```python
from build123d import *

# Parameters (mm, degrees)
BOSS_EXTRUDE3_DEPTH                           = 12.7
BOSS_EXTRUDE4_DEPTH                           = 38.1
CBORE_FOR_M3_PAN_HEAD_MACHINE_SCREW1_AT_COUNT = 2
CBORE_FOR_M3_PAN_HEAD_MACHINE_SCREW1_AT_PITCH = 66.51875294
CBORE_FOR_M3_PAN_HEAD_MACHINE_SCREW1_2_COUNT  = 2
CBORE_FOR_M3_PAN_HEAD_MACHINE_SCREW1_2_PITCH  = 66.51875294


with BuildPart() as part:
    # Sketch1 → Boss-Extrude3 (new body)
    with BuildSketch(Plane(origin=(0, 0, 0), x_dir=(0, 0, -1), z_dir=(1, 0, 0))):
        with BuildLine():
            Line((38.1, -76.2), (38.1, 0))
            ThreePointArc((38.1, 0), (0, 38.1), (-38.1, 0))
            Line((-38.1, 0), (-38.1, -76.2))
            Line((-38.1, -76.2), (38.1, -76.2))
        make_face()
    extrude(amount=BOSS_EXTRUDE3_DEPTH)

    # Sketch5 → Boss-Extrude4 (add)
    with BuildSketch(Plane(origin=(12.7, 0, 0), x_dir=(0, 0, -1), z_dir=(1, 0, 0))):
        with BuildLine():
            ThreePointArc((-20.358389677, 0), (0, 20.358389677), (20.358389677, 0))
            Line((20.358389677, 0), (38.1, 0))
            ThreePointArc((38.1, 0), (0, 38.1), (-38.1, 0))
            Line((-38.1, 0), (-20.358389677, 0))
        make_face()
    extrude(amount=BOSS_EXTRUDE4_DEPTH)

    # Sketch8 → CBORE for M3 Pan Head Machine Screw1 (revolve, cut)
    with BuildSketch(Plane(origin=(12.7, 0, 0), x_dir=(0, 0, -1), z_dir=(0, 1, 0))):
        Polygon((0, 0), (0, 12.7), (1.7, 12.7), (1.7, 2.4), (3.5, 2.4), (3.5, 0.025), (3.525, 0), align=None)
    cbore_for_m3_pan_head_machine_screw1 = revolve(axis=Axis((19.05, 0, 0), (-1, 0, 0)), mode=Mode.SUBTRACT)

    # CBORE for M3 Pan Head Machine Screw1 at: CBORE for M3 Pan Head Machine Screw1 ×2
    with Locations(*[Vector(0, -0.924225465, 0.381847207) * (i * CBORE_FOR_M3_PAN_HEAD_MACHINE_SCREW1_AT_PITCH) for i in range(1, CBORE_FOR_M3_PAN_HEAD_MACHINE_SCREW1_AT_COUNT)]):
        add(cbore_for_m3_pan_head_machine_screw1, mode=Mode.SUBTRACT)

    # CBORE for M3 Pan Head Machine Screw1 2: CBORE for M3 Pan Head Machine Screw1 ×2
    with Locations(*[Vector(0, -0.924225465, -0.381847207) * (i * CBORE_FOR_M3_PAN_HEAD_MACHINE_SCREW1_2_PITCH) for i in range(1, CBORE_FOR_M3_PAN_HEAD_MACHINE_SCREW1_2_COUNT)]):
        add(cbore_for_m3_pan_head_machine_screw1, mode=Mode.SUBTRACT)


solid = part.part
```
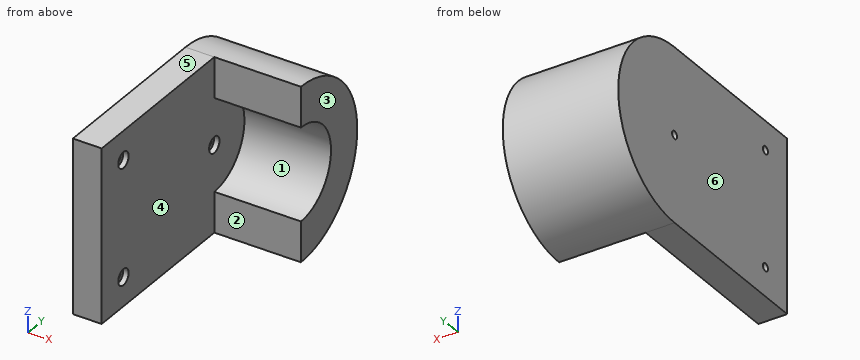
CAD build for the part. Positions are in the model's coordinates, mm. Face numbers are marked on the shaded views. A direction names the side the tool comes from. Coordinates: 2 decimals unless noted, no trailing zeros. Write each loop counter-clockwise with the first axis right and the second up, starting at its lowest first coordinate (ties: lowest second). Pieces come first, ordered by that corner, then holes. Notation, with made-up numbers: (-5.5, 65.5) -> (14.5, 65.5) arc R30 ccw to (14.5, 89.5) -> close; hole circle Ø3 at (3, 72). An arc over 180 degrees is marked (long way). Return JSON: item names as keys, results as strings. Group by question number.
Q1. Which spindle directions (+Z, -Z, +X, -X, +Y, -Y) get a long thin tool onto all of the face, cutting with end or side? Do the marked faces 1, 2 and 3. Say none if no direction does.
Q2. Cut at D-D, the plane z = -25.4. Give the cut face in (x, y) (3 decimals), then the cut area to 3 significant figures.
Q3. Cut at B-B, the plane y = 10.5. Give the cut face in (x, z).
Q4. Cut at C-C, the plane x = 4.5. Give the cut face in (y, z), then the cut area to 3 significant figures.
Q5. Flat gauge pins, fed straight in: pin 1 (4 mm diameter, centred on y = -46.5, z = -18, fed in from +X); pin 2 (3.5 mm diameter, centred on y = -60.5, z = 25.5, fed in from +X); pin 3 (8 mm diameter, centred on y = -61.48, z = -25.4, fed in from -X); pin 4 (14 mm diameter, centred on x = 34, z = -25, fed in from -Y). Where does each tip first touch, or does it go through?
Q6. Drill centre lines: line 1 (Z direction, x = 5, y = 0); line 2 (X direction, y = -41.5, z = -11.5); line 3 (Z direction, x = 10, y = -62.5). Where is each one in solid material? Low to high.
Q7. Pull direction X, two halves, no side cores. Call the marked faces 4, 5 and 6: released by +X, released by -X, zero draft, split by the parting line, or undercut.
Q8. Cut at A-A, the plane z = 0. Give the cut face in (x, y) (3 decimals).
Returned:
{
 "1": {"face 1": "+X, -Y", "face 2": "+Z, -Z, +X, -Y", "face 3": "+Z, -Z, +X, +Y, -Y"},
 "2": {"outline": "(0, -76.2) -> (12.7, -76.2) -> (12.7, -65.003) -> (12.675, -64.978) -> (10.3, -64.978) -> (10.3, -63.178) -> (0, -63.178) -> close; (0, -59.778) -> (10.3, -59.778) -> (10.3, -57.978) -> (12.675, -57.978) -> (12.7, -57.953) -> (12.7, 0) -> (50.8, 0) -> (50.8, 28.398) -> (0, 28.398) -> close", "area": "2,360 mm2"},
 "3": {"outline": "(0, -36.62) -> (50.8, -36.62) -> (50.8, -17.44) -> (12.7, -17.44) -> (12.7, 17.44) -> (50.8, 17.44) -> (50.8, 36.62) -> (0, 36.62) -> close"},
 "4": {"outline": "(-76.2, -38.1) -> (0, -38.1) arc R38.1 ccw to (0, 38.1) -> (-76.2, 38.1) -> close; hole circle Ø3.4 at (-61.48, -25.4); hole circle Ø3.4 at (-61.48, 25.4); hole circle Ø3.4 at (0, 0)", "area": "8,060 mm2"},
 "5": {"pin 1": "stops at x = 12.7", "pin 2": "stops at x = 10.3", "pin 3": "stops at x = 0", "pin 4": "stops at y = 0"},
 "6": {"line 1": "z = -38.1 to -1.7, 1.7 to 38.1", "line 2": "x = 0 to 12.7", "line 3": "z = -38.1 to -26.76, -24.04 to 24.04, 26.76 to 38.1"},
 "7": {"face 4": "released by +X", "face 5": "zero draft", "face 6": "released by -X"},
 "8": {"outline": "(0, -76.2) -> (12.7, -76.2) -> (12.7, -3.525) -> (12.675, -3.5) -> (10.3, -3.5) -> (10.3, -1.7) -> (0, -1.7) -> close; (0, 1.7) -> (10.3, 1.7) -> (10.3, 3.5) -> (12.675, 3.5) -> (12.7, 3.525) -> (12.7, 20.358) -> (50.8, 20.358) -> (50.8, 38.1) -> (0, 38.1) -> close"}
}
